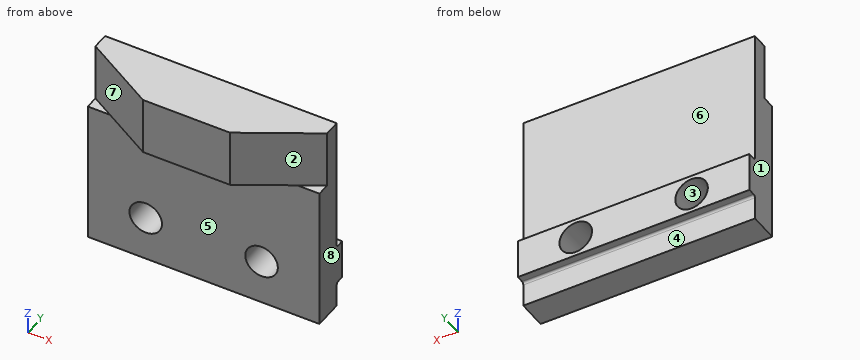
from build123d import *

# Parameters (mm, degrees)
SKETCH1_W           = 50.8
SKETCH1_H           = 44.45
BOSS_EXTRUDE1_DEPTH = 3.175
BOSS_EXTRUDE2_START = -3.175
SKETCH2_W           = 50.8
SKETCH2_H           = 12.7
BOSS_EXTRUDE2_DEPTH = 6.35
BOSS_EXTRUDE3_START = 3.175
SKETCH3_W           = 50.8
SKETCH3_H           = 8.7376
BOSS_EXTRUDE3_DEPTH = 2.032
CUT_EXTRUDE2_START  = 22.225
CUT_EXTRUDE2_DEPTH  = 12.7
CUT_EXTRUDE4_START  = 22.225
CUT_EXTRUDE4_DEPTH  = 12.7
CUT_EXTRUDE6_START  = 5.207
SKETCH6_R           = 3.5687
CUT_EXTRUDE6_DEPTH  = 9.525
FILLET1_R           = 0.508


with BuildPart() as part:
    # Sketch1 → Boss-Extrude1 (new, symmetric)
    with BuildSketch(Plane(origin=(0, 0, 0), x_dir=(1, 0, 0), z_dir=(0, 1, 0))):
        Rectangle(SKETCH1_W, SKETCH1_H)
    extrude(amount=BOSS_EXTRUDE1_DEPTH, both=True)

    # Sketch2 → Boss-Extrude2 (add)
    with BuildSketch(Plane(origin=(0, 0, 0), x_dir=(1, 0, 0), z_dir=(0, 1, 0)).offset(BOSS_EXTRUDE2_START)):
        with Locations((0, -15.875)):
            Rectangle(SKETCH2_W, SKETCH2_H)
    extrude(amount=-BOSS_EXTRUDE2_DEPTH)

    # Sketch3 → Boss-Extrude3 (add)
    with BuildSketch(Plane(origin=(0, 0, 0), x_dir=(1, 0, 0), z_dir=(0, 1, 0)).offset(BOSS_EXTRUDE3_START)):
        with Locations((0, 12.319)):
            Rectangle(SKETCH3_W, SKETCH3_H)
    extrude(amount=BOSS_EXTRUDE3_DEPTH)

    # Sketch4 → Cut-Extrude2 (cut)
    with BuildSketch(Plane.XY.offset(CUT_EXTRUDE2_START)):
        Polygon((-76.2, -22.225), (-9.525, -22.225), (-9.525, -9.525), (-76.2, 28.969829198), align=None)
    extrude(amount=-CUT_EXTRUDE2_DEPTH, mode=Mode.SUBTRACT)

    # Sketch5 → Cut-Extrude4 (cut)
    with BuildSketch(Plane.XY.offset(CUT_EXTRUDE4_START)):
        Polygon((9.525, -22.225), (76.2, -22.225), (76.2, 28.969829198), (9.525, -9.525), align=None)
    extrude(amount=-CUT_EXTRUDE4_DEPTH, mode=Mode.SUBTRACT)

    # Sketch6 → Cut-Extrude6 (cut)
    with BuildSketch(Plane(origin=(0, 0, 0), x_dir=(1, 0, 0), z_dir=(0, 1, 0)).offset(CUT_EXTRUDE6_START)):
        with Locations(Location((-12.7, 12.319, 0), (0, 0, 270))):
            Circle(SKETCH6_R)
        with Locations(Location((12.7, 12.319, 0), (0, 0, 270))):
            Circle(SKETCH6_R)
    extrude(amount=-CUT_EXTRUDE6_DEPTH, mode=Mode.SUBTRACT)

    # Fillet1
    fillet1_edges = [part.edges().sort_by_distance(p)[0] for p in [
        (0, 3.175, -7.9502),
        (0, 3.175, -16.6878),
    ]]
    fillet(fillet1_edges, radius=FILLET1_R)


solid = part.part
Work out the finished part from the listing and answer in its coordinate system (mm). Face numbers are marked on the shaded views. A direction names the side the tool comes from. Coordinates: 2 decimals unless noted, no trailing zeros. Order: outer loops, then holes, each group sorted by start corner. A loop starts at its lowest first (then second) coordinate and runs counter-clockwise, first axis right, second up. Notation, with made-up numbers: (40.5, 89) - (55.5, 89) arc R23 ccw to (55.5, 101) - close; hole circle Ø4 at (65, 51). An arc over 180 degrees is marked (long way). Put each result on its own line as item: value. Start each with the question number.
1) Flat-ended cylindrical pins translate along their axes: pin 1 (6 mm diameter, centred on x = -12, z = 16, fed in from +Y) (3 decimals); pin 2 (11.5 mm diameter, centred on x = -12.7, z = -12.319, fed in from -Y) (3 decimals); pin 3 (8 mm diameter, centred on x = -10, y = -6.5, fed in from -Z) (3 decimals); pin 4 (0.8 mm diameter, centred on x = -10, y = 4, fed in from +Z). Find the tip coordinate at first contact, or state that the pin passes through.
2) Find the intervals of material crossed by line 1 (X direction, y = -2, z = -14); line 2 (Y direction, x = 5.5, z = -9) (3 decimals); line 3 (Y direction, x = 2.5, z = 7) (3 decimals), in increasing order. Write a range as from..to.
3) For a pull along X with two mould halves and no side action, classify the marked faces 1, 2, 3 and 4 as released by +X, released by -X, zero draft, split by the parting line, or undercut.
4) Find section A-A (x = 14). Give the vertices of the cut face in (y, z) (1 decimal).
5) Find section B-B (z = -13). Give the vertices of the cut face in (x, y) (3 decimals), plus the area to 3 significant figures.
6) For the marked faces 5, 6, 7 and 8, determine the directions among +Z, -Z, +X, -X, +Y, -Y from which every point of the face is accessible in a straight line to the end or side of a thin tool.
7) Find section D-D (x = 3.5). Give the vertices of the cut face in (y, z) (3 decimals), plus the area to 3 significant figures.
8) Find section C-C (y = -1). Give the vertices of the cut face in (x, z) (3 decimals).
Results list:
1. pin 1: stops at y = 3.175
1. pin 2: stops at y = -3.175
1. pin 3: stops at z = -22.225
1. pin 4: stops at z = -7.94
2. line 1: x = -25.4..-15.85, -9.55..9.55, 15.85..25.4
2. line 2: y = -3.175..5.207
2. line 3: y = -3.175..3.175
3. face 1: released by -X
3. face 2: released by +X
3. face 3: undercut
3. face 4: zero draft
4. outline: (-6.9, 9.5) - (-3.2, 9.5) - (-3.2, -9) - (5.2, -9) - (5.2, -8) - (3.7, -8) arc R0.5 cw to (3.2, -7.4) - (3.2, 22.2) - (-6.9, 22.2) - close; (-3.2, -22.2) - (3.2, -22.2) - (3.2, -17.2) arc R0.5 cw to (3.7, -16.7) - (5.2, -16.7) - (5.2, -15.6) - (-3.2, -15.6) - close
5. outline: (-25.4, -3.175) - (-16.203, -3.175) - (-16.203, 5.207) - (-25.4, 5.207) - close; (-9.197, -3.175) - (9.197, -3.175) - (9.197, 5.207) - (-9.197, 5.207) - close; (16.203, -3.175) - (25.4, -3.175) - (25.4, 5.207) - (16.203, 5.207) - close
5. area: 308 mm^2
6. face 5: -Z, +X, -X, -Y
6. face 6: +Z, +X, -X, +Y
6. face 7: +Z, -X, -Y
6. face 8: +Z, -Z, +X, +Y, -Y
7. outline: (-9.525, 9.525) - (-3.175, 9.525) - (-3.175, -22.225) - (3.175, -22.225) - (3.175, -17.196) arc R0.508 cw to (3.683, -16.688) - (5.207, -16.688) - (5.207, -7.95) - (3.683, -7.95) arc R0.508 cw to (3.175, -7.442) - (3.175, 22.225) - (-9.525, 22.225) - close
7. area: 381 mm^2
8. outline: (-25.4, -22.225) - (25.4, -22.225) - (25.4, 9.525) - (24.291, 9.525) - (24.291, 22.225) - (-24.291, 22.225) - (-24.291, 9.525) - (-25.4, 9.525) - close; hole circle Ø7.137 at (-12.7, -12.319); hole circle Ø7.137 at (12.7, -12.319)
